Study the drawing (mm; zero at the part's minimum x, y, z) and answer. Round coordinates to 2 decimals unless told otherwise and drop trailing zeros. Order: outer loops, then holes, each group sorted by start corner. A loop starts at its lowest first (then second) coordinate and runs counter-clockwise, first axis right, second up. Notation, with made-up numbers: (3.25, 46) - (42.25, 46) arc R11 cw to (42.25, 67) - close; hole circle Ø7 at (-24, -31). An arc over 180 degrees is marked (long way). Use one line per item in the form item = value. Start each with the question number.
Q1. For a pull along X with two mould halves and no side action, classify the marked faces 1, 2 and 3 as +X half, -X half, draft (parallel to the pull), parting line (faces both ways), or undercut.
Q2. Given P1, Ø1.5, axis at x = 22, y = 3.5, coming from the -Z side; P2, Ø2, axis at x = 24, y = 6, coming from the -Z side; P3, Ø3, axis at x = 9, z = 15.5, coming from the +Y side; P4, Ø12, axis at x = 4, z = 20, coming from the -Y side, each flat-ended and moving along its own axis, determine where each tip first touches the part or whether it passes through.
Q3. The part is cut by section A-A on y = 9. Determine the outline of the cut face in (x, z) (3 decimals), plus the area to 3 significant figures.
Q4. Find the intervals of material crossed by line 1 (Z direction, x = 14.25, y = 1.5); line 2 (Y direction, x = 13.5, z = 2); line 3 (X direction, y = 7.5, z = 5.5), in increasing order. Write a range as [from, to].
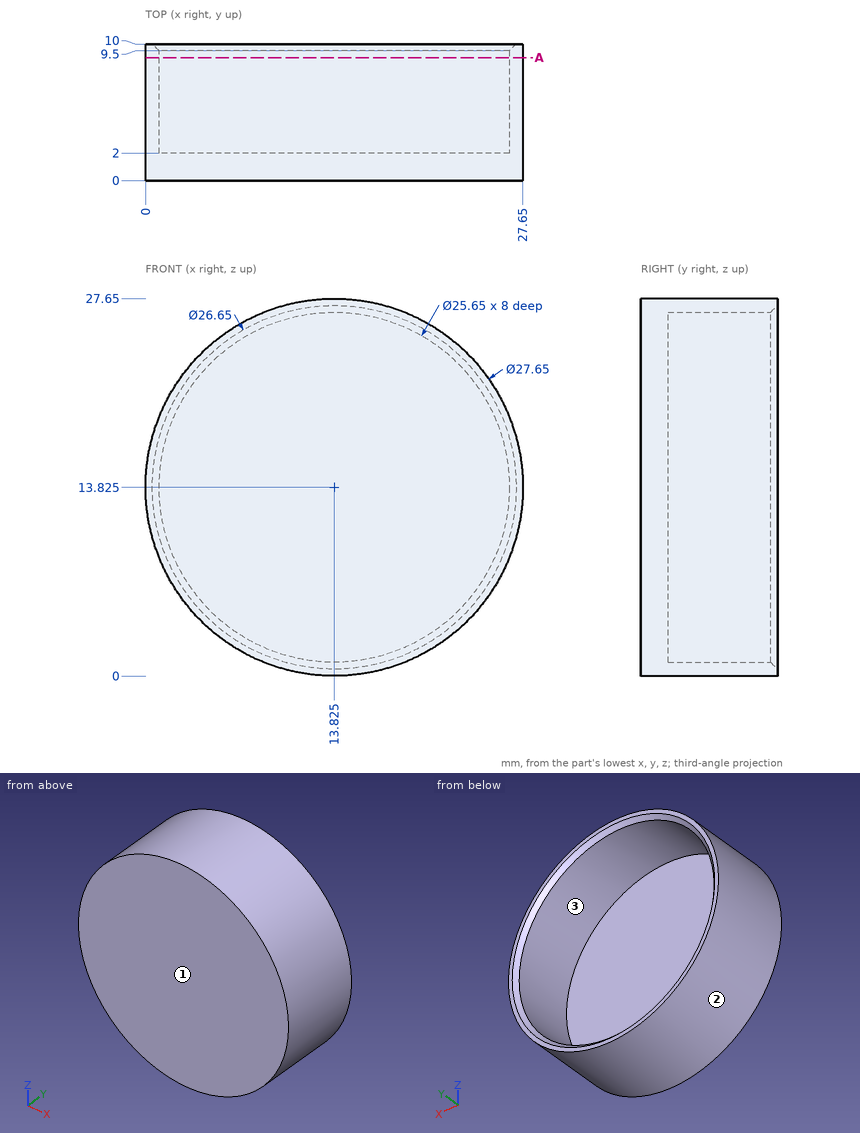
Found:
q1.face_1 = draft
q1.face_2 = parting line
q1.face_3 = undercut
q2.P1 = 2.16
q2.P2 = 3.48
q2.P3 = 2
q2.P4 = 0
q3.outline = circle Ø27.65 at (13.825, 13.825); hole circle Ø25.65 at (13.825, 13.825)
q3.area = 83.7 mm²
q4.line_1 = [0.01, 27.64]
q4.line_2 = [0, 2]
q4.line_3 = [2.79, 4.07], [23.58, 24.86]
